```python
from build123d import *

# Parameters (mm, degrees)
SKETCH1_R           = 0.75
BOSS_EXTRUDE1_DEPTH = 2


with BuildPart() as part:
    # Sketch1 → Boss-Extrude1 (new body)
    with BuildSketch(Plane.XY):
        with BuildLine():
            Line((16.2, 4), (16.2, 2))
            ThreePointArc((16.2, 2), (15.614213562, 0.585786438), (14.2, 0))
            Line((14.2, 0), (2, 0))
            ThreePointArc((2, 0), (0.585786438, 0.585786438), (0, 2))
            Line((0, 2), (0, 4))
            Line((0, 4), (4, 4))
            Line((4, 4), (4, 6))
            Line((4, 6), (0, 6))
            Line((0, 6), (0, 8.645))
            Line((0, 8.645), (4, 8.645))
            Line((4, 8.645), (4, 10.645))
            Line((4, 10.645), (0, 10.645))
            Line((0, 10.645), (0, 12.645))
            ThreePointArc((0, 12.645), (0.585786438, 14.059213562), (2, 14.645))
            Line((2, 14.645), (14.2, 14.645))
            ThreePointArc((14.2, 14.645), (15.614213562, 14.059213562), (16.2, 12.645))
            Line((16.2, 12.645), (16.2, 10.645))
            Line((16.2, 10.645), (12.2, 10.645))
            Line((12.2, 10.645), (12.2, 8.645))
            Line((12.2, 8.645), (16.2, 8.645))
            Line((16.2, 8.645), (16.2, 6))
            Line((16.2, 6), (12.2, 6))
            Line((12.2, 6), (12.2, 4))
            Line((12.2, 4), (16.2, 4))
        make_face()
        with Locations((13.45, 2.5)):
            Circle(SKETCH1_R, mode=Mode.SUBTRACT)
        with Locations((2.75, 12.145)):
            Circle(SKETCH1_R, mode=Mode.SUBTRACT)
        with Locations((13.45, 12.145)):
            Circle(SKETCH1_R, mode=Mode.SUBTRACT)
        with Locations((2.75, 2.5)):
            Circle(SKETCH1_R, mode=Mode.SUBTRACT)
    extrude(amount=BOSS_EXTRUDE1_DEPTH)


solid = part.part
```
Read the model definition and answer for the solid it produces. Units are mm, in the model's axes. A direction names the side the tool comes from. Round coordinates to 2 decimals unless told otherwise and drop trailing zeros. Write each loop counter-clockwise with the first axis right and the second up, starting at its lowest first coordinate (ties: lowest second). Pieces come first, ordered by that corner, then holes. Notation, with made-up numbers: (64.5, 22.5) -> (68.5, 22.5) arc R30 ccw to (68.5, 54.5) -> close; hole circle Ø10 at (-33, 81). An arc over 180 degrees is marked (long way). Answer in a Markdown table with one row per item. Add a question column.
1) Consider line 1 (Y direction, x = 13.45, z = 1.15) (3 decimals); line 2 (Y direction, x = 1.75, z = 0.55) (3 decimals); line 3 (X direction, y = 9.5, z = 1.3). Determine where each line is inside the solid, lowest interval first.
2) Find section B-B, the plane x = 13.45. Determine the outline of the cut face in (y, z) (3 decimals), and give its area (3 significant figures).
3) Determine the mould class of faces 4 (the face through (2.155, 2.044, 0.986)), 5 (the face through (16.2, 3, 1)), 6 (the face through (0.57, 14.044, 0.986)) for opening direction Y: pulls with the +Y half, pulls with the -Y half, needs draft (parallel to the pull), parting line crosses it, or undercut.
4) Find section A-A, the plane y = 2.5. Determine the outline of the cut face in (x, z), and give its area (3 significant figures).
5) Which of the six approach directions +Z, -Z, +X, -X, +Y, -Y give full straight-line access (tool end or side, diameter ignored) to faces 1 (the face through (14, 6, 1)), 2 (the face through (2, 10.645, 1)), 3 (the face through (0, 7, 1))?
6) Find section D-D, the plane y = 5.5. Determine the outline of the cut face in (x, z), and give its area (3 significant figures).
7) Find section C-C, the plane z = 1.7. Determine the outline of the cut face in (x, y) (3 decimals).
8) Given P1, Ø1.2, axis at x = 2.75, y = 2.5, coming from the -Z side, flat-ended and moving along its own axis, determine where the tip first touches the part or whether it passes through.
Findings below:
| question | item | result |
|---|---|---|
| 1 | line 1 | 0 to 1.75, 3.25 to 4, 6 to 8.645, 10.645 to 11.395, 12.895 to 14.645 |
| 1 | line 2 | 0.016 to 4, 6 to 8.645, 10.645 to 14.629 |
| 1 | line 3 | 4 to 12.2 |
| 2 | outline | (0, 0) -> (1.75, 0) -> (1.75, 2) -> (0, 2) -> close; (3.25, 0) -> (4, 0) -> (4, 2) -> (3.25, 2) -> close; (6, 0) -> (8.645, 0) -> (8.645, 2) -> (6, 2) -> close; (10.645, 0) -> (11.395, 0) -> (11.395, 2) -> (10.645, 2) -> close; (12.895, 0) -> (14.645, 0) -> (14.645, 2) -> (12.895, 2) -> close |
| 2 | area | 15.3 mm² |
| 3 | face 4 | undercut |
| 3 | face 5 | needs draft |
| 3 | face 6 | pulls with the +Y half |
| 4 | outline | (0, 0) -> (2, 0) -> (2, 2) -> (0, 2) -> close; (3.5, 0) -> (12.7, 0) -> (12.7, 2) -> (3.5, 2) -> close; (14.2, 0) -> (16.2, 0) -> (16.2, 2) -> (14.2, 2) -> close |
| 4 | area | 26.4 mm² |
| 5 | face 1 | +Z, -Z, +X |
| 5 | face 2 | +Z, -Z, -X |
| 5 | face 3 | +Z, -Z, -X, +Y, -Y |
| 6 | outline | (4, 0) -> (12.2, 0) -> (12.2, 2) -> (4, 2) -> close |
| 6 | area | 16.4 mm² |
| 7 | outline | (0, 2) arc R2 ccw to (2, 0) -> (14.2, 0) arc R2 ccw to (16.2, 2) -> (16.2, 4) -> (12.2, 4) -> (12.2, 6) -> (16.2, 6) -> (16.2, 8.645) -> (12.2, 8.645) -> (12.2, 10.645) -> (16.2, 10.645) -> (16.2, 12.645) arc R2 ccw to (14.2, 14.645) -> (2, 14.645) arc R2 ccw to (0, 12.645) -> (0, 10.645) -> (4, 10.645) -> (4, 8.645) -> (0, 8.645) -> (0, 6) -> (4, 6) -> (4, 4) -> (0, 4) -> close; hole circle Ø1.5 at (2.75, 2.5); hole circle Ø1.5 at (2.75, 12.145); hole circle Ø1.5 at (13.45, 2.5); hole circle Ø1.5 at (13.45, 12.145) |
| 8 | P1 | through |
